from build123d import *

# Parameters (mm, degrees)
SKETCH2_W           = 76.2
SKETCH2_H           = 76.2
BOSS_EXTRUDE1_DEPTH = 2.54
SKETCH7_R           = 1.7145
CUT_EXTRUDE1_DEPTH  = 5.08
SKETCH9_W           = 4.572
SKETCH9_H           = 25.4
CUT_EXTRUDE2_DEPTH  = 5.08
SKETCH6_R           = 2.794
CUT_EXTRUDE3_DEPTH  = 5.08


with BuildPart() as part:
    # Sketch2 → Boss-Extrude1 (new body)
    with BuildSketch(Plane.XY):
        Rectangle(SKETCH2_W, SKETCH2_H)
    extrude(amount=BOSS_EXTRUDE1_DEPTH)

    # Sketch7 → Cut-Extrude1 (cut)
    with BuildSketch(Plane(origin=(0, 0, 0), x_dir=(-1, 0, 0), z_dir=(0, 0, -1))):
        with Locations((25.278322628, -17.651318113)):
            Circle(SKETCH7_R)
        with Locations((25.278322628, 33.148681887)):
            Circle(SKETCH7_R)
        with Locations((-25.521677372, 33.148681887)):
            Circle(SKETCH7_R)
        with Locations((-25.521677372, -17.651318113)):
            Circle(SKETCH7_R)
    extrude(amount=-CUT_EXTRUDE1_DEPTH, mode=Mode.SUBTRACT)

    # Sketch9 → Cut-Extrude2 (cut)
    with BuildSketch(Plane.XY.offset(2.54)):
        with Locations((8.023665405, 0)):
            Rectangle(SKETCH9_W, SKETCH9_H)
        with Locations((-8.023665405, 0)):
            Rectangle(SKETCH9_W, SKETCH9_H)
    extrude(amount=-CUT_EXTRUDE2_DEPTH, mode=Mode.SUBTRACT)

    # Sketch6 → Cut-Extrude3 (cut)
    with BuildSketch(Plane(origin=(0, 0, 0), x_dir=(-1, 0, 0), z_dir=(0, 0, -1))):
        with Locations((33.02, 33.02)):
            Circle(SKETCH6_R)
        with Locations((-33.02, 33.02)):
            Circle(SKETCH6_R)
        with Locations((-33.02, -33.02)):
            Circle(SKETCH6_R)
        with Locations((33.02, -33.02)):
            Circle(SKETCH6_R)
    extrude(amount=-CUT_EXTRUDE3_DEPTH, mode=Mode.SUBTRACT)


solid = part.part
CAD build for the part. Positions are in the model's coordinates, mm. A direction names the side the tool comes from. Round coordinates to 2 decimals unless told otherwise and drop trailing zeros. Write each loop counter-clockwise with the first axis right and the second up, starting at its lowest first coordinate (ties: lowest second). Pieces come first, ordered by that corner, then holes. Notation, with made-up numbers: M 7.25,30 L 61.25,30 A6 ccw 61.25,34 Z; hole C 58,22 d1. An arc over 180 degrees is marked long. Use a Markdown table: item, result. Add a question column.
1. Flat gauge pin, fed straight in: P1, Ø2.5, axis at x = 25.52, y = -17.65, coming from the +Z side. Where does the tip first touch, or does it go through?
2. 3-axis set-ups, long thin cutter, end or side, ignore diameter. For faces 1 (the face through (-1, 1, 2.54)), 2 (the face through (5.738, 0, 1)): which of +Z, -Z, +X, -X, +Y, -Y reach the whole face in a straight line?
3. Pull direction Y, two halves, no side cores. Call faces 3 (the face through (-1, 1, 0)), 4 (the face through (-1, 38.1, 1)), 5 (the face through (35.08, -31.13, 1.25)): released by +Y, released by -Y, zero draft, split by the parting line, or undercut.
4. Slice it at C-C on z = 0.5. Give the number of separate pieces and of enclosed holes in the cut face, then the cut area to 3 significant figures.
5. Drill centre lines: probe 1 along Y at (x, z) = (-33.02, 2.05); probe 2 along Y at (x, z) = (25.5, 1.5); probe 3 along X at (y, z) = (12, 1.9). Where is each one in solid material? Low to high.
6. Slice it at A-A on x = 33.02. Give the cut face in (y, z).
Reply:
| question | item | result |
|---|---|---|
| 1 | P1 | passes through |
| 2 | face 1 | +Z, +X, -X, +Y, -Y |
| 2 | face 2 | +Z, -Z |
| 3 | face 3 | zero draft |
| 3 | face 4 | released by +Y |
| 3 | face 5 | undercut |
| 4 | separate pieces | 1 |
| 4 | enclosed holes | 10 |
| 4 | area | 5,440 mm^2 |
| 5 | probe 1 | y = -38.1 to -35.81, -30.23 to 30.23, 35.81 to 38.1 |
| 5 | probe 2 | y = -38.1 to -19.37, -15.94 to 31.43, 34.86 to 38.1 |
| 5 | probe 3 | x = -38.1 to -10.31, -5.74 to 5.74, 10.31 to 38.1 |
| 6 | outline | M -38.1,0 L -35.81,0 L -35.81,2.54 L -38.1,2.54 Z; M -30.23,0 L 30.23,0 L 30.23,2.54 L -30.23,2.54 Z; M 35.81,0 L 38.1,0 L 38.1,2.54 L 35.81,2.54 Z |
